Source: CAD feature listing. Evaluate the final solid. Frame: model axes, mm. Face numbers are marked on the shaded views. A direction names the side the tool comes from. Coordinates: 2 decimals unless noted, no trailing zeros. Order: outer loops, then holes, each group sorted by start corner. A loop starts at its lowest first (then second) coordinate and runs counter-clockwise, first axis right, second up. Notation, with made-up numbers: (53.5, -38.75) - (87.5, -38.75) arc R7 ccw to (87.5, -31.75) - close; hole circle Ø4 at (-5, 71). An arc over 180 degrees is marked (long way). One line per question, with ' | ' between items. Start each with the question number.
(1) Section A-A (x = 2.25). Return the cut outline in (y, z).
(2) Contact query for flat-ended pins moving along their axis: P1, Ø1.6, axis at x = 23.18, y = -1.71, coming from the +Z side; P2, Ø1, axis at x = 8, z = -1, coming from the -Y side; P3, Ø1.4, axis at x = 2.57, z = -3.78, coming from the -Y side; P4, Ø1.9, axis at x = 23.11, z = -4.56, coming from the +Y side. Output: stop coordinate, or through.
(3) Section B-B (z = -4). Return the cut outline in (x, y).
(4) Line query: line 1 along Y through (x, z) = (8.25, -2); line 2 along Z through (x, y) = (21, -2.5). Output: solid intervals per line, ascending.
(5) Access query for the marked faces 1, 2 and 3. Directions: +Z, -Z, +X, -X, +Y, -Y. A direction counts if a zero-diameter tool reaches every point of the face in a straight line with its end or side. Return the directions, or none.
(6) Section C-C (x = 7.25). Return the cut outline in (y, z), then the cut area to 3 significant figures.
(7) Section D-D (z = -1.25). Return the cut outline in (x, y), then the cut area to 3 significant figures.
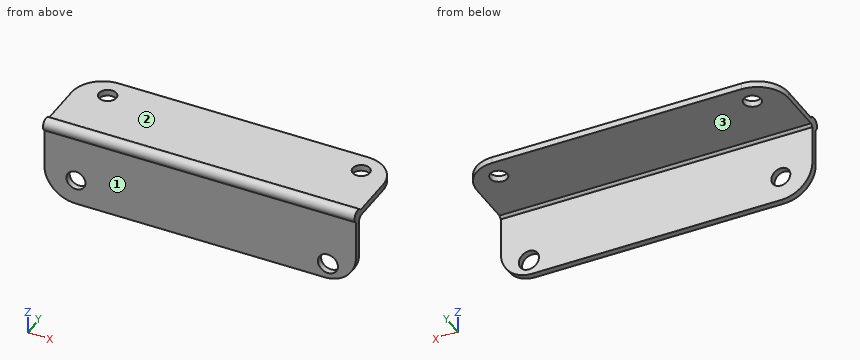
from build123d import *

# Parameters (mm, degrees)
BOSS_EXTRUDE1_DEPTH = 0.508
BOSS_EXTRUDE2_DEPTH = 0.508
SKETCH3_R           = 0.508
BOSS_EXTRUDE3_DEPTH = 25.4
SKETCH4_R           = 0.694806542
SKETCH4_R_2         = 0.705318585
CUT_EXTRUDE1_DEPTH  = 25.4
SKETCH5_R           = 0.773137268
SKETCH5_R_2         = 0.818403862
CUT_EXTRUDE2_DEPTH  = 25.4


with BuildPart() as part:
    # Sketch1 → Boss-Extrude1 (new body)
    with BuildSketch(Plane.XY):
        with BuildLine():
            Line((2.54, 0), (22.86, 0))
            ThreePointArc((22.86, 0), (24.656051224, -0.743948776), (25.4, -2.54))
            Line((25.4, -2.54), (25.4, -6.35))
            Line((25.4, -6.35), (0, -6.35))
            Line((0, -6.35), (0, -2.54))
            ThreePointArc((0, -2.54), (0.743948776, -0.743948776), (2.54, 0))
        make_face()
    extrude(amount=BOSS_EXTRUDE1_DEPTH)

    # Sketch2 → Boss-Extrude2 (add)
    with BuildSketch(Plane.XZ.offset(6.35)):
        with BuildLine():
            Line((25.4, 0.508), (0, 0.508))
            Line((0, 0.508), (0, -3.302))
            ThreePointArc((0, -3.302), (0.743948776, -5.098051224), (2.54, -5.842))
            Line((2.54, -5.842), (22.86, -5.842))
            ThreePointArc((22.86, -5.842), (24.656051224, -5.098051224), (25.4, -3.302))
            Line((25.4, -3.302), (25.4, 0.508))
        make_face()
    extrude(amount=BOSS_EXTRUDE2_DEPTH)

    # Sketch3 → Boss-Extrude3 (add)
    with BuildSketch(Plane(origin=(25.4, 0, 0), x_dir=(0, 0, -1), z_dir=(1, 0, 0))):
        with Locations((-0.257183831, -6.571194295)):
            Circle(SKETCH3_R)
    extrude(amount=-BOSS_EXTRUDE3_DEPTH)

    # Sketch4 → Cut-Extrude1 (cut)
    with BuildSketch(Plane(origin=(0, 0, 0), x_dir=(-1, 0, 0), z_dir=(0, 0, -1))):
        with Locations((-23.184832038, -1.708481591)):
            Circle(SKETCH4_R)
        with Locations((-2.513571979, -1.708481591)):
            Circle(SKETCH4_R_2)
    extrude(amount=-CUT_EXTRUDE1_DEPTH, mode=Mode.SUBTRACT)

    # Sketch5 → Cut-Extrude2 (cut)
    with BuildSketch(Plane(origin=(0, -6.35, 0), x_dir=(1, 0, 0), z_dir=(0, 1, 0))):
        with Locations(Location((2.571816613, 3.784683683, 0), (0, 0, 270))):
            Circle(SKETCH5_R)
        with Locations(Location((23.109034226, 4.557820951, 0), (0, 0, 270))):
            Circle(SKETCH5_R_2)
    extrude(amount=-CUT_EXTRUDE2_DEPTH, mode=Mode.SUBTRACT)


solid = part.part
Response values:
1) outline: (-6.86, -5.83) - (-6.35, -5.83) - (-6.35, -4.49) - (-6.86, -4.49) - close; (-6.86, -3.08) - (-6.35, -3.08) - (-6.35, -0.2) arc R0.51 ccw to (-6.13, 0) - (-2.36, 0) - (-2.36, 0.51) - (-6.13, 0.51) arc R0.51 ccw (long way) to (-6.86, -0.16) - close; (-1.05, 0) - (-0.02, 0) - (-0.02, 0.51) - (-1.05, 0.51) - close
2) P1: stops at z = 0.51 | P2: stops at y = -6.86 | P3: passes through | P4: stops at y = -6.35
3) outline: (0.1, -6.86) - (1.83, -6.86) - (1.83, -6.35) - (0.1, -6.35) - close; (3.31, -6.86) - (22.51, -6.86) - (22.51, -6.35) - (3.31, -6.35) - close; (23.71, -6.86) - (25.3, -6.86) - (25.3, -6.35) - (23.71, -6.35) - close
4) line 1: y = -6.86 to -6.35 | line 2: z = 0 to 0.51
5) face 1: -Z, +X, -X, -Y | face 2: +Z, +X, -X, +Y | face 3: -Z, +X, -X, +Y
6) outline: (-6.86, -5.84) - (-6.35, -5.84) - (-6.35, -0.2) arc R0.51 ccw to (-6.13, 0) - (0, 0) - (0, 0.51) - (-6.13, 0.51) arc R0.51 ccw (long way) to (-6.86, -0.16) - close | area: 6.75 mm²
7) outline: (0, -6.86) - (25.4, -6.86) - (25.4, -6.35) - (0, -6.35) - close | area: 12.9 mm²
